For this review, take the finished solid that the model builds, in its own axes (mm). A direction names the side the tool comes from. Round coordinates to 2 decimals unless told otherwise and drop trailing zeros. Order: outer loops, then holes, each group sorted by start corner. A loop starts at its lowest first (then second) coordinate and runs counter-clockwise, first axis right, second up. Notation, with made-up numbers: (-6.75, 35) -> (52.25, 35) arc R18 ccw to (52.25, 70) -> close; hole circle Ø3 at (73.25, 83). An arc over 180 degrees is marked (long way). Answer in a Markdown table with one row per item.
Autodesk Inventor part; units mm, degrees
ref_plane "YZ Plane" through (0, 0, 0) normal (1, 0, 0) x (0, 1, 0)
ref_plane "XZ Plane" through (0, 0, 0) normal (0, 1, 0) x (-1, 0, 0)
ref_plane "XY Plane" through (0, 0, 0) normal (0, 0, 1) x (1, 0, 0)
sketch "Sketch1" plane through (0, 0, 0) normal (0, 1, 0) x (-1, 0, 0)
  line L0 (0, 0) -> (-70, 0)
  line L1 (-70, 0) -> (-70, -60)
  line L2 (-70, -60) -> (0, -60)
  line L3 (0, -60) -> (0, 0)
  line L4 (0, -60) -> (0, -77.7966)
  line L5 (0, -77.7966) -> (-70, -60)
  dimension "d0" = 70
  dimension "d1" = 60
  dimension "d23" = 14.264
extrude "Extrusion1" add sketch "Sketch1" along normal blind 3
sketch "Sketch3" plane through (0, 3, 0) normal (0, 1, 0) x (1, 0, 0)
  circle A0 centre (67.75, 20.25) radius 1.25
  circle A1 centre (67.75, 29.75) radius 1.25
  line L0 (70, 0) -> (70, 60)
  line L1 (0, 0) -> (70, 0)
  line L2 (6, 10) -> (9, 10)
  line L3 (9, 10) -> (9, 16)
  line L4 (9, 16) -> (6, 16)
  line L5 (6, 16) -> (6, 10)
  line L6 (6, 37) -> (9, 37)
  line L7 (9, 37) -> (9, 31)
  line L8 (9, 31) -> (6, 31)
  line L9 (6, 31) -> (6, 37)
  line L10 (0, 77.7966) -> (0, 0)
  dimension "d15" = 2.5
  dimension "d16" = 2.25
  dimension "d17" = 2.25
  dimension "d18" = 2.5
  dimension "d19" = 20.25
  dimension "d20" = 9.5
  dimension "d24" = 3
  dimension "d25" = 6
  dimension "d26" = 6
  dimension "d27" = 10
  dimension "d28" = 15
  dimension "d29" = 6
extrude "Extrusion3" cut sketch "Sketch3" along normal through all both and the other way through all
equation "\"d17\" = d16"
equation "\"d18\" = d15"
properties part number "pinball-case-left-wall-outer-scaled"
Q1. Take a section at B-B, the plane y = 1.85. Write out the cut boundary in (x, z).
Answer key:
| item | result |
|---|---|
| outline | (0, -77.8) -> (70, -60) -> (70, 0) -> (0, 0) -> close; hole (6, -37) -> (9, -37) -> (9, -31) -> (6, -31) -> close; hole (6, -16) -> (9, -16) -> (9, -10) -> (6, -10) -> close; hole circle Ø2.5 at (67.75, -29.75); hole circle Ø2.5 at (67.75, -20.25) |
Q2. Tool access review of faces 4 (the face through (70, 1, -30)), 5 (the face through (8, 2, -16)): name each direction out of +Z, -Z, +X, -X, +Y, -Y from which nothing blocks a thin tool from reaching the whole face with its end or side.
Answer key:
| item | result |
|---|---|
| face 4 | +Z, -Z, +X, +Y, -Y |
| face 5 | +Y, -Y |
Q3. Take a section at A-A, the plane z = -29.75. Write out the cut boundary in (x, y).
Answer key:
| item | result |
|---|---|
| outline | (0, 0) -> (66.5, 0) -> (66.5, 3) -> (0, 3) -> close; (69, 0) -> (70, 0) -> (70, 3) -> (69, 3) -> close |
Q4. Take a section at C-C, the plane x = 67.75. Write out the cut boundary in (y, z).
Answer key:
| item | result |
|---|---|
| outline | (0, -60.57) -> (3, -60.57) -> (3, -31) -> (0, -31) -> close; (0, -28.5) -> (3, -28.5) -> (3, -21.5) -> (0, -21.5) -> close; (0, -19) -> (3, -19) -> (3, 0) -> (0, 0) -> close |
Q5. The part is to be moulded in two halves that separate along Z. For faces 1 (the face through (35, 1, 0)), 2 (the face through (6, 2, -34)), 3 (the face through (34.51, 1.479, -69.023)), say which applies: +Z half, -Z half, draft (parallel to the pull), parting line (faces both ways), or undercut.
Answer key:
| item | result |
|---|---|
| face 1 | +Z half |
| face 2 | undercut |
| face 3 | -Z half |
Q6. Take a section at D-D, the plane z = -14. Write out the cut boundary in (x, y).
Answer key:
| item | result |
|---|---|
| outline | (0, 0) -> (6, 0) -> (6, 3) -> (0, 3) -> close; (9, 0) -> (70, 0) -> (70, 3) -> (9, 3) -> close |
Q7. To check wall thickness, follow probe 1 along X at (y, z) = (2.1, -29.75); probe 2 along Z at (x, y) = (67.75, 0.7); probe 3 along Z at (x, y) = (48, 2.1). State the ranges of each line that lie inside material, in increasing order.
Answer key:
| item | result |
|---|---|
| probe 1 | x = 0 to 66.5, 69 to 70 |
| probe 2 | z = -60.57 to -31, -28.5 to -21.5, -19 to 0 |
| probe 3 | z = -65.59 to 0 |
